Build history of the part. All positions in model axes, mm. Face numbers are marked on the shaded views. Give positions to 0.01 mm unless a question says otherwise; leave off trailing zeros. Write each loop counter-clockwise with the first axis right and the second up, starting at its lowest first coordinate (ties: lowest second). Pieces come first, ordered by that corner, then holes. Notation, with made-up numbers: (-23.75, -1.5) -> (-17.75, -1.5) arc R19 ccw to (-17.75, 10.5) -> close; hole circle Ø7 at (-7, 62). An arc over 180 degrees is marked (long way). Put each result on its own line as item: value. Start each with the question number.
Item 1: Drill centre lines: line 1 along Z through (x, y) = (-29, -0.65); line 2 along Y through (x, z) = (21, 29); line 3 along X through (y, z) = (-1, -17.5). Where is each one in solid material? Low to high.
Item 2: Slice it at A-A, the plane x = -29. List the corners of the cut face in (y, z), plus the area to 3 significant figures.
Item 3: Slice it at B-B, the plane z = -29. List the corners of the cut face in (x, y).
Item 4: Flat gauge pins, fed straight in: pin 1 Ø5 at (y, z) = (-6, 23.5) entering from -X; pin 2 Ø2 at (x, z) = (28.5, -15.5) entering from -Y; pin 3 Ø1 at (x, z) = (16.5, 13.5) entering from -Y; pin 4 Ø7.5 at (x, y) = (25.5, -4.5) entering from +Z. Where does each tip first touch, or does it go through?
Item 5: Slice it at D-D, the plane z = 20. List the corners of the cut face in (x, y).
Item 6: Two-plate mould, pull along Y, no slides. Class the marked faces 1, 2, 3 and 4: pulls with the +Y half, pulls with the -Y half, needs draft (parallel to the pull), parting line crosses it, or undercut.
Item 7: Slice it at C-C, the plane y = -4.5. List the corners of the cut face in (x, z), plus the area to 3 significant figures.
```python
from build123d import *

# Parameters (mm, degrees)
F0_W     = 64
F0_H     = 64
F0_R     = 1.5
F1_DEPTH = 1.4
F2_W     = 20
F2_H     = 20
F2_R     = 7.65
F3_DEPTH = 6
F4_DEPTH = 21
F2_W_2   = 6.7
F2_H_2   = 13.9
F5_DEPTH = 7
F6_W     = 4
F6_H     = 5
F7_DEPTH = 8.9


with BuildPart() as f1:
    # F0 (on Front) → F1 (new body)
    with BuildSketch(Plane.XZ):
        Rectangle(F0_W, F0_H)
        with Locations((-29, -29)):
            Circle(F0_R, mode=Mode.SUBTRACT)
        with Locations((29, -29)):
            Circle(F0_R, mode=Mode.SUBTRACT)
        with Locations((-29, 29)):
            Circle(F0_R, mode=Mode.SUBTRACT)
        with Locations((29, 29)):
            Circle(F0_R, mode=Mode.SUBTRACT)
    extrude(amount=F1_DEPTH)

    # F2 (on face) → F3 (join)
    with BuildSketch(Plane.XZ.offset(1.4)):
        with Locations((0, 20)):
            Rectangle(F2_W, F2_H)
        with Locations((0, 20)):
            Circle(F2_R, mode=Mode.SUBTRACT)
    extrude(amount=F3_DEPTH)

    # F4 (add): a face of the model
    f4_faces = [f1.faces().sort_by_distance(p)[0] for p in [
        (0, -1.4, 20),
    ]]
    extrude(f4_faces, amount=F4_DEPTH)

    # F2 (on face) → F5 (join)
    with BuildSketch(Plane.XZ.offset(1.4)):
        with Locations((27.15, -15.15)):
            Rectangle(F2_W_2, F2_H_2)
    extrude(amount=F5_DEPTH)

    # F6 (on face) → F7 (join)
    with BuildSketch(Plane.YZ.offset(30.5)):
        with Locations((-5.6, -17.7)):
            Rectangle(F6_W, F6_H)
    extrude(amount=F7_DEPTH)


solid = f1.part
```
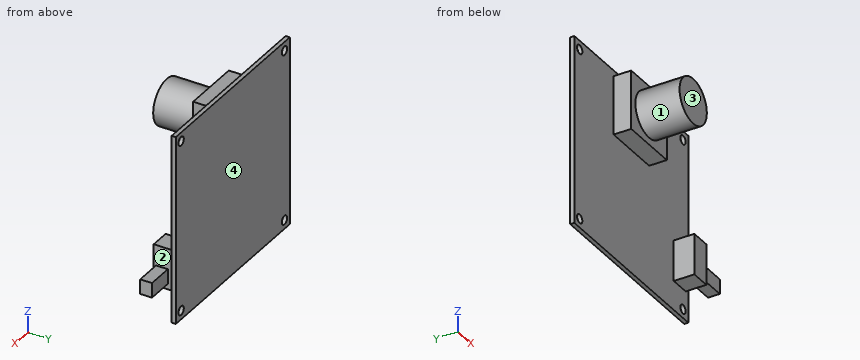
Values follow:
1. line 1: -32 to -30.5, -27.5 to 27.5, 30.5 to 32
1. line 2: -1.4 to 0
1. line 3: -32 to 32
2. outline: (-1.4, -32) -> (0, -32) -> (0, -30.5) -> (-1.4, -30.5) -> close; (-1.4, -27.5) -> (0, -27.5) -> (0, 27.5) -> (-1.4, 27.5) -> close; (-1.4, 30.5) -> (0, 30.5) -> (0, 32) -> (-1.4, 32) -> close
2. area: 81.2 mm2
3. outline: (-32, -1.4) -> (-30.5, -1.4) -> (-30.5, 0) -> (-32, 0) -> close; (-27.5, -1.4) -> (27.5, -1.4) -> (27.5, 0) -> (-27.5, 0) -> close; (30.5, -1.4) -> (32, -1.4) -> (32, 0) -> (30.5, 0) -> close
4. pin 1: x = -10
4. pin 2: y = -8.4
4. pin 3: y = -1.4
4. pin 4: z = 32
5. outline: (-32, -1.4) -> (-10, -1.4) -> (-10, -7.4) -> (-7.65, -7.4) -> (-7.65, -22.4) -> (7.65, -22.4) -> (7.65, -7.4) -> (10, -7.4) -> (10, -1.4) -> (32, -1.4) -> (32, 0) -> (-32, 0) -> close
6. face 1: needs draft
6. face 2: undercut
6. face 3: pulls with the -Y half
6. face 4: pulls with the +Y half
7. outline: (-10, 10) -> (10, 10) -> (10, 30) -> (-10, 30) -> close; (23.8, -22.1) -> (30.5, -22.1) -> (30.5, -20.2) -> (39.4, -20.2) -> (39.4, -15.2) -> (30.5, -15.2) -> (30.5, -8.2) -> (23.8, -8.2) -> close
7. area: 538 mm2
